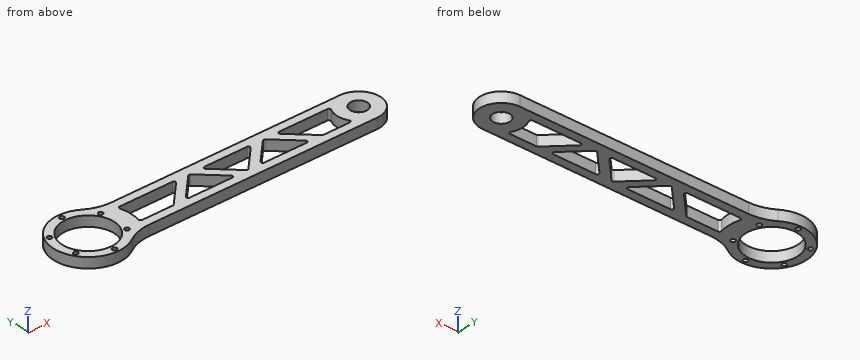
```python
from build123d import *

# Parameters (mm, degrees)
EXTRUDE_1_DEPTH         = 12
SKETCH_5_R              = 30
SKETCH_5_R_2            = 10
CUT_EXTRUDE_1_DEPTH     = 348.51834484
CUT_EXTRUDE_3_DEPTH     = 348.51834484
FILLET_1_R              = 2
HOLE_WIZARD_5_2_5_2_1_D = 5.2


with BuildPart() as part:
    # 草图1 → 凸台-拉伸1 (new body)
    with BuildSketch(Plane.XY):
        with BuildLine():
            Line((320, 25), (49.749371855, 25))
            ThreePointArc((49.749371855, 25), (35.315615126, 27.128644612), (22.110831936, 33.333333333))
            ThreePointArc((22.110831936, 33.333333333), (-40, 0), (22.110831936, -33.333333333))
            ThreePointArc((22.110831936, -33.333333333), (35.315615126, -27.128644612), (49.749371855, -25))
            Line((49.749371855, -25), (320, -25))
            ThreePointArc((320, -25), (345, 0), (320, 25))
        make_face()
    extrude(amount=EXTRUDE_1_DEPTH)

    # 草图5 → 切除-拉伸1 (cut, through all)
    with BuildSketch(Plane.XY.offset(12)):
        Circle(SKETCH_5_R)
        with Locations((320, 0)):
            Circle(SKETCH_5_R_2)
    extrude(amount=-CUT_EXTRUDE_1_DEPTH, mode=Mode.SUBTRACT)

    # 草图6 → 切除-拉伸3 (cut, through all)
    with BuildSketch(Plane.XY.offset(12)):
        with BuildLine():
            Line((47.696960071, 15), (117.696960071, 15))
            Line((117.696960071, 15), (87.696960071, -15))
            Line((87.696960071, -15), (47.696960071, -15))
            ThreePointArc((47.696960071, -15), (50, 0), (47.696960071, 15))
        make_face()
        Polygon((131.839095695, 15), (101.839095695, -15), (161.839095695, -15), align=None)
        Polygon((145.981231318, 15), (175.981231318, -15), (205.981231318, 15), align=None)
        Polygon((220.123366942, 15), (190.123366942, -15), (250.123366942, -15), align=None)
        with BuildLine():
            Line((234.265502566, 15), (264.265502566, -15))
            Line((264.265502566, -15), (300, -15))
            ThreePointArc((300, -15), (295, 0), (300, 15))
            Line((300, 15), (234.265502566, 15))
        make_face()
    extrude(amount=-CUT_EXTRUDE_3_DEPTH, mode=Mode.SUBTRACT)

    # 圆角1
    fillet_1_edges = [part.edges().sort_by_distance(p)[0] for p in [
        (117.696960071, 15, 6),
        (87.696960071, -15, 6),
        (47.696960071, -15, 6),
        (47.696960071, 15, 6),
        (145.981231318, 15, 6),
        (205.981231318, 15, 6),
        (175.981231318, -15, 6),
        (300, 15, 6),
        (300, -15, 6),
        (264.265502566, -15, 6),
        (234.265502566, 15, 6),
        (220.123366942, 15, 6),
        (250.123366942, -15, 6),
        (190.123366942, -15, 6),
        (131.839095695, 15, 6),
        (161.839095695, -15, 6),
        (101.839095695, -15, 6),
    ]]
    fillet(fillet_1_edges, radius=FILLET_1_R)

    # Ø5.2 (5.2) 直径孔1 (through all)
    with Locations(Plane(origin=(0, 35, 12), x_dir=(1, 0, 0), z_dir=(0, 0, 1))):
        with Locations((0, 0), (-30.310889132, -17.5), (-30.310889132, -52.5), (0, -70), (30.310889132, -52.5), (30.310889132, -17.5)):
            Hole(HOLE_WIZARD_5_2_5_2_1_D / 2)


solid = part.part
```
Work out the finished part from the listing and answer in its coordinate system (mm). Coordinates: 2 decimals unless noted, no trailing zeros. Write each loop counter-clockwise with the first axis right and the second up, starting at its lowest first coordinate (ties: lowest second). Pieces come first, ordered by that corner, then holes.
Q1. A cutting plane is placed at D-D, the plane x = 215. Give the vertices of the cut face in (y, z), then the cut area to 3 significant figures.
Q2. Find the intervals of material crossed by line 1 (Y direction, x = 0, z = 9); line 2 (X direction, y = -14.5, z = 4.75); line 3 (Y direction, x = 320, z = 9.25), in increasing order.
Q3. A cutting plane is placed at A-A, the plane x = 68.5. Give the vertices of the cut face in (y, z).
Q4. Each of these flat-tipped pins is pushed along its axis until it touches: pin 1 Ø1 at (x, z) = (31, 1.5) entering from +Y; pin 2 Ø6 at (x, z) = (210, 3.5) entering from +Y; pin 3 Ø1 at (x, z) = (27.5, 7.5) entering from -Y. Where does it stop, or does it pass through?
Q5. A cutting plane is placed at B-B, the plane y = 0. State how many separate pieces and enclosed holes the cut face has, then the cut area to 3 significant figures.
Findings below:
1. outline: (-25, 0) - (-15, 0) - (-15, 12) - (-25, 12) - close; (9.88, 0) - (25, 0) - (25, 12) - (9.88, 12) - close
1. area: 301 mm2
2. line 1: y = -40 to -37.6, -32.4 to -30, 30 to 32.4, 37.6 to 40
2. line 2: x = -37.28 to -26.26, 26.26 to 49.03, 88.19 to 105.34, 158.33 to 193.63, 246.62 to 263.77, 297.66 to 340.37
2. line 3: y = -25 to -10, 10 to 25
3. outline: (-25, 0) - (-15, 0) - (-15, 12) - (-25, 12) - close; (15, 0) - (25, 0) - (25, 12) - (15, 12) - close
4. pin 1: stops at y = 28.85
4. pin 2: stops at y = 25
4. pin 3: stops at y = -30.48
5. separate pieces: 8
5. enclosed holes: 0
5. area: 1,400 mm2
